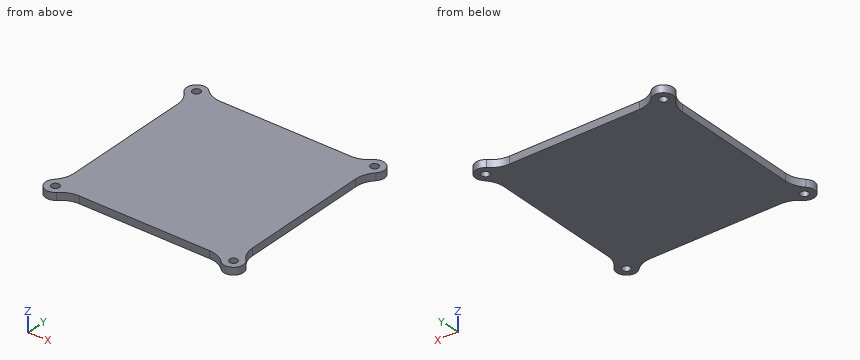
```python
from build123d import *

# Parameters (mm, degrees)
SKETCH_1_R      = 1.625
EXTRUDE_1_DEPTH = 3
FILLET_1_R      = 10


with BuildPart() as part:
    # Эскиз1 → Бобышка-Вытянуть1 (new body)
    with BuildSketch(Plane.XY):
        with BuildLine():
            ThreePointArc((-36.516055554, -32.516055554), (-39.344482678, -39.344482678), (-32.516055554, -36.516055554))
            Line((-32.516055554, -36.516055554), (32.516055554, -36.516055554))
            ThreePointArc((32.516055554, -36.516055554), (39.344482678, -39.344482678), (36.516055554, -32.516055554))
            Line((36.516055554, -32.516055554), (36.516055554, 32.516055554))
            ThreePointArc((36.516055554, 32.516055554), (39.344482678, 39.344482678), (32.516055554, 36.516055554))
            Line((32.516055554, 36.516055554), (-32.516055554, 36.516055554))
            ThreePointArc((-32.516055554, 36.516055554), (-39.344482678, 39.344482678), (-36.516055554, 32.516055554))
            Line((-36.516055554, 32.516055554), (-36.516055554, -32.516055554))
        make_face()
        with Locations((-36.516055554, -36.516055554)):
            Circle(SKETCH_1_R, mode=Mode.SUBTRACT)
        with Locations((36.516055554, 36.516055554)):
            Circle(SKETCH_1_R, mode=Mode.SUBTRACT)
        with Locations((-36.516055554, 36.516055554)):
            Circle(SKETCH_1_R, mode=Mode.SUBTRACT)
        with Locations((36.516055554, -36.516055554)):
            Circle(SKETCH_1_R, mode=Mode.SUBTRACT)
    extrude(amount=EXTRUDE_1_DEPTH)

    # Скругление1
    fillet_1_edges = [part.edges().sort_by_distance(p)[0] for p in [
        (-36.516055554, -32.516055554, 1.5),
        (-36.516055554, 32.516055554, 1.5),
        (-32.516055554, 36.516055554, 1.5),
        (32.516055554, 36.516055554, 1.5),
        (36.516055554, 32.516055554, 1.5),
        (36.516055554, -32.516055554, 1.5),
        (32.516055554, -36.516055554, 1.5),
        (-32.516055554, -36.516055554, 1.5),
    ]]
    fillet(fillet_1_edges, radius=FILLET_1_R)


solid = part.part
```
Can you work these out from the model? Positions are in its coordinate system, mm. Give positions to 0.01 mm unless a question says otherwise; leave off trailing zeros. Loops run counter-clockwise (first coordinate to the right, second up) from the corner with the lowest first, then second, coordinate; pieces in that order, holes last. Notation, with made-up numbers: M 49,82 L 62,82 A31 cw 62,116 Z; hole C 11.5,69 d2. An arc over 180 degrees is marked long. Use one line per item in the form item = value. Start each with the question number.
(1) I want a section at B-B, the plane y = 18. Write out the boundary of the cut face in (x, z).
(2) I want a section at A-A, the plane z = 0.75. Write out the boundary of the cut face in (x, y) (3 decimals).
(3) Please list where these lines run through material, in increasing order: line 1 (X direction, y = 37.5, z = 0.45); line 2 (X direction, y = 4, z = 1.7).
(4) I'm going to push flat-ended pins straight in: P1, Ø1, axis at x = -8, z = 2, coming from the +Y side; P2, Ø1, axis at x = 22.5, z = 1, coming from the -Y side. Where does each tip first touch, or does it pass through?
Worked out:
q1.outline = M -36.52,0 L 36.52,0 L 36.52,3 L -36.52,3 Z
q2.outline = M -39.373,-33.717 A4 ccw -33.717,-39.373 A10 cw -26.718,-36.516 L 26.718,-36.516 A10 cw 33.717,-39.373 A4 ccw 39.373,-33.717 A10 cw 36.516,-26.718 L 36.516,26.718 A10 cw 39.373,33.717 A4 ccw 33.717,39.373 A10 cw 26.718,36.516 L -26.718,36.516 A10 cw -33.717,39.373 A4 ccw -39.373,33.717 A10 cw -36.516,26.718 L -36.516,-26.718 A10 cw Z; hole C -36.516,-36.516 d3.25; hole C -36.516,36.516 d3.25; hole C 36.516,-36.516 d3.25; hole C 36.516,36.516 d3.25
q3.line_1 = -40.39 to -37.81, -35.22 to -31.04, 31.04 to 35.22, 37.81 to 40.39
q3.line_2 = -36.52 to 36.52
q4.P1 = 36.52
q4.P2 = -36.52
